from build123d import *

# Parameters (mm, degrees)
F0_R     = 3.175
F1_DEPTH = 3.048


with BuildPart() as f1:
    # F0 (on Front) → F1 (new body)
    with BuildSketch(Plane.XZ):
        with BuildLine():
            ThreePointArc((3.175, 0), (-2.2450640303, -2.2450640303), (0, 3.175))
            Line((0, 3.175), (0, 9.525))
            ThreePointArc((0, 9.525), (-6.7351920908, 6.7351920908), (-9.525, 0))
            ThreePointArc((-9.525, 0), (-6.7351920908, -6.7351920908), (0, -9.525))
            Line((0, -9.525), (0.6773435479, -9.500885786))
            ThreePointArc((0.6773435479, -9.500885786), (6.9705567315, -6.4912990883), (9.525, 0))
            Line((9.525, 0), (3.175, 0))
        make_face()
        with BuildLine():
            ThreePointArc((-9.525, 0), (-6.7351920908, 6.7351920908), (0, 9.525))
            Line((0, 9.525), (0, 47.625))
            ThreePointArc((0, 47.625), (-10.644756084, 51.722700101), (-15.7942028036, 61.9003804205))
            Line((-15.7942028036, 61.9003804205), (-9.525, 0))
        make_face()
        with BuildLine():
            Line((0, 47.625), (0, 9.525))
            ThreePointArc((0, 9.525), (6.7351920908, 6.7351920908), (9.525, 0))
            Line((9.525, 0), (36.5125, 0))
            ThreePointArc((36.5125, 0), (38.8373399243, 5.6126600757), (44.45, 7.9375))
            Line((44.45, 7.9375), (23.8252, 7.9375))
            ThreePointArc((23.8252, 7.9375), (18.2035596682, 10.2660596682), (15.875, 15.8877))
            Line((15.875, 15.8877), (15.875, 63.5))
            ThreePointArc((15.875, 63.5), (11.2253201513, 52.2746798487), (0, 47.625))
        make_face()
        with BuildLine():
            Line((36.5125, 0), (9.525, 0))
            ThreePointArc((9.525, 0), (6.9705567315, -6.4912990883), (0.6773435479, -9.500885786))
            Line((0.6773435479, -9.500885786), (44.7324052746, -7.9324746146))
            ThreePointArc((44.7324052746, -7.9324746146), (38.9380895153, -5.7116327839), (36.5125, 0))
        make_face()
        with BuildLine():
            ThreePointArc((-15.7942028036, 61.9003804205), (-10.644756084, 51.722700101), (0, 47.625))
            Line((0, 47.625), (0, 60.325))
            ThreePointArc((0, 60.325), (-3.175, 63.5), (0, 66.675))
            Line((0, 66.675), (0, 79.375))
            ThreePointArc((0, 79.375), (-10.5003255158, 75.40625), (-15.7504882737, 65.484375))
            ThreePointArc((-15.7504882737, 65.484375), (-15.8738192656, 63.6936154008), (-15.7942028036, 61.9003804205))
        make_face()
        with BuildLine():
            Line((0, 60.325), (0, 47.625))
            ThreePointArc((0, 47.625), (11.2253201513, 52.2746798487), (15.875, 63.5))
            ThreePointArc((15.875, 63.5), (15.8430821396, 64.5061676396), (15.7474569047, 65.5082893304))
            ThreePointArc((15.7474569047, 65.5082893304), (10.4912828548, 75.4142187767), (0, 79.375))
            Line((0, 79.375), (0, 66.675))
            ThreePointArc((0, 66.675), (2.2450640303, 65.7450640303), (3.175, 63.5))
            ThreePointArc((3.175, 63.5), (2.2450640303, 61.2549359697), (0, 60.325))
        make_face()
        with BuildLine():
            ThreePointArc((44.45, 7.9375), (38.8373399243, 5.6126600757), (36.5125, 0))
            ThreePointArc((36.5125, 0), (38.9380895153, -5.7116327839), (44.7324052746, -7.9324746146))
            ThreePointArc((44.7324052746, -7.9324746146), (50.1616327839, -5.5119104847), (52.3875, 0))
            ThreePointArc((52.3875, 0), (50.0626600757, 5.6126600757), (44.45, 7.9375))
        make_face()
        with BuildLine():
            ThreePointArc((47.625, 0), (44.45, -3.175), (41.275, 0))
            ThreePointArc((41.275, 0), (44.45, 3.175), (47.625, 0))
        make_face(mode=Mode.SUBTRACT)
        with BuildLine():
            ThreePointArc((0, -9.525), (0.3388863295, -9.5189695375), (0.6773435479, -9.500885786))
            Line((0.6773435479, -9.500885786), (0, -9.525))
        make_face()
        with BuildLine():
            Line((-9.4502929642, 115.490625), (-15.7504882737, 65.484375))
            ThreePointArc((-15.7504882737, 65.484375), (-10.5003255158, 75.40625), (0, 79.375))
            Line((0, 79.375), (0, 104.775))
            ThreePointArc((0, 104.775), (-7.14375, 107.9998046905), (-9.4502929642, 115.490625))
        make_face()
        with Locations((-6.4251534641, 100.4420816898)):
            Circle(F0_R, mode=Mode.SUBTRACT)
        with BuildLine():
            ThreePointArc((0, 79.375), (10.4912828548, 75.4142187767), (15.7474569047, 65.5082893304))
            Line((15.7474569047, 65.5082893304), (9.525, 114.3))
            ThreePointArc((9.525, 114.3), (6.7351920908, 107.5648079092), (0, 104.775))
            Line((0, 104.775), (0, 79.375))
        make_face()
        with BuildLine():
            ThreePointArc((9.525, 114.3), (0.596483242, 123.8063048942), (-9.4502929642, 115.490625))
            ThreePointArc((-9.4502929642, 115.490625), (-7.14375, 107.9998046905), (0, 104.775))
            ThreePointArc((0, 104.775), (6.7351920908, 107.5648079092), (9.525, 114.3))
        make_face()
        with BuildLine():
            ThreePointArc((3.175, 114.3), (2.2450640303, 112.0549359697), (0, 111.125))
            ThreePointArc((0, 111.125), (-2.2450640303, 116.5450640303), (3.175, 114.3))
        make_face(mode=Mode.SUBTRACT)
        with BuildLine():
            Line((0, 9.525), (0, 3.175))
            ThreePointArc((0, 3.175), (2.2450640303, 2.2450640303), (3.175, 0))
            Line((3.175, 0), (9.525, 0))
            ThreePointArc((9.525, 0), (6.7351920908, 6.7351920908), (0, 9.525))
        make_face()
    extrude(amount=F1_DEPTH)


solid = f1.part
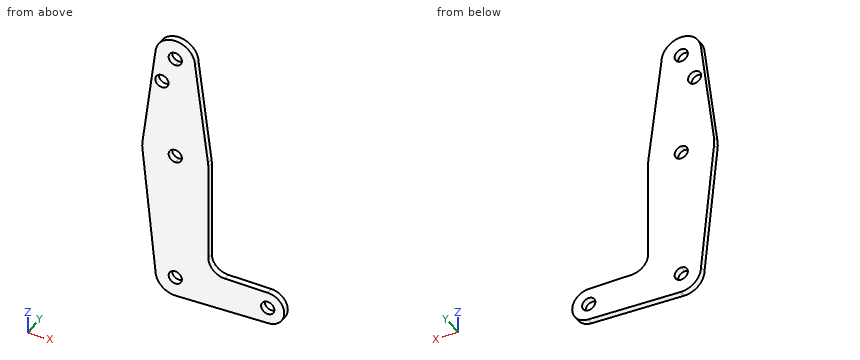
Source: CAD feature listing. Evaluate the final solid. Frame: model axes, mm. Coordinates: 2 decimals unless noted, no trailing zeros. Loops run counter-clockwise (first coordinate to the right, second up) from the corner with the lowest first, then second, coordinate; pieces in that order, holes last. Notation, with made-up numbers: M -17,87 L -10,87 A25 cw -10,121 Z; hole C 67,80.5 d10. An arc over 180 degrees is marked long. Answer in a Markdown table with one row per item.
Q1. First-contact query: pin 1 (10 mm diameter, centred on x = -6.43, z = 100.44, fed in from +Y); pin 2 (1.5 mm diameter, centred on y = -2, z = 32, fed in from +X) (3 decimals). Flat tips, straight axial feed; report the tip coordinate or a pass-through.
Answers below:
| item | result |
|---|---|
| pin 1 | stops at y = 0 |
| pin 2 | stops at x = 15.875 |
Q2. Section A-A on y = -1.5. State how many separate pieces and enclosed holes the cut face has, plus the area to 3 significant figures.
Answers below:
| item | result |
|---|---|
| separate pieces | 1 |
| enclosed holes | 5 |
| area | 3,900 mm^2 |
Q3. Section C-C on z = 22.5. Return the cut outline in (x, y) (3 decimals), plus the area to 3 significant figures.
Answers below:
| item | result |
|---|---|
| outline | M -11.804,-3.048 L 15.875,-3.048 L 15.875,0 L -11.804,0 Z |
| area | 84.4 mm^2 |
Q4. Section B-B on x = 7. Return the cut outline in (y, z), plus the area to 3 significant figures.
Answers below:
| item | result |
|---|---|
| outline | M -3.05,-9.28 L 0,-9.28 L 0,120.76 L -3.05,120.76 Z |
| area | 396 mm^2 |
Q5. Ray query, probe 1 along Z at (x, y) = (0, -0.6) (3 decimals); probe 2 along X at (y, z) = (-1.2, 114.3) (3 decimals); probe 3 along X at (y, z) = (-0.9, -1.5). Return the intervals inside material, ascending. Write a range as from..to.
Answers below:
| item | result |
|---|---|
| probe 1 | z = -9.525..-3.175, 3.175..60.325, 66.675..111.125, 117.475..123.825 |
| probe 2 | x = -9.6..-3.175, 3.175..9.525 |
| probe 3 | x = -9.41..-2.8, 2.8..41.65, 47.25..52.24 |
